Input: part model. Units: mm. Frame: model coordinates. Face numbers are marked on the shaded views. A direction names the side the tool comes from. Give positions to 0.01 mm unless a question says otherwise; leave off trailing zeros. Write each loop counter-clockwise with the first axis right and the second up, starting at its lowest first coordinate (ties: lowest second). Pieces come first, ordered by that corner, then holes. Notation, with made-up numbers: (-20.5, 2) - (-13.5, 2) arc R23 cw to (-13.5, 14) - close; hole circle Ø8 at (86.5, -12). An arc over 180 degrees is marked (long way). Use a Markdown table: item, result. Add a question column.
1. Mould query, pull axis Y, two halves, no side actions, for the marked faces 1, 2, 3 and 4. Classes: released by +Y, released by -Y, zero draft, split by the parting line, or undercut.
2. Material intervals for probe 1 along X at (y, z) = (49, -14); probe 2 along Y at (x, z) = (78.5, 1); probe 3 along Z at (x, y) = (32.5, 46), sorted ascending.
3. Section query C-C, the plane z = -5.5. Return loops of the section in (x, y).
4. Pin query (flat end, axial travel): pin 1 (1.5 mm diameter, centred on x = 49.5, y = 40, fed in from +Z); pin 2 (1 mm diameter, centred on x = 102.5, y = 47.5, fed in from -Z); pin 3 (12 mm diameter, centred on x = 31, z = -10.5, fed in from +Y). Return the tip coordinate at first contact, or that it passes through.
5. Section query B-B, the plane x = 82. Return loops of the section in (y, z), plus the area to 3 significant figures.
6. Set-up query: the marked faces 5, 6 and 7. Return all of +Z, -Z, +X, -X, +Y, -Y with unobstructed straight access to the full face (end or side cutting, diameter ignored); none if empty.
7. Section query D-D, the plane x = 6. Return loops of the section in (y, z).
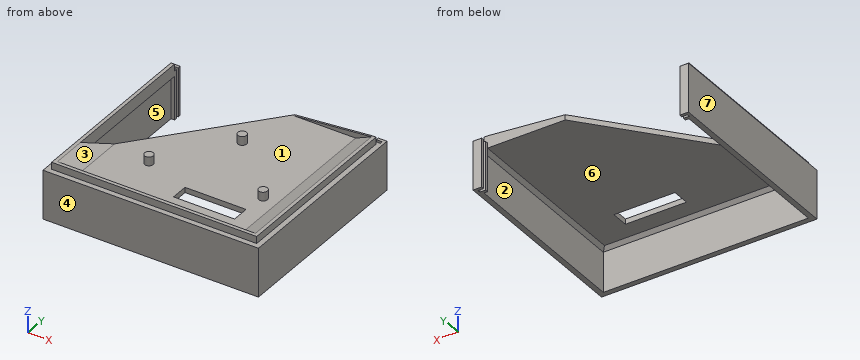
Autodesk Fusion 360 part; units mm, degrees
sketch "Sketch1" plane through (0, 0, 0) normal (0, 0, 1) x (1, 0, 0)
  line L0 (0, 0) -> (113.6, 0)
  line L1 (113.6, 0) -> (113.6, 101.8)
  line L2 (113.6, 101.8) -> (0, 101.8)
  line L3 (0, 101.8) -> (0, 0)
  line L4 (-2, -2) -> (115.6, -2)
  line L5 (115.6, -2) -> (115.6, 103.8)
  line L6 (115.6, 103.8) -> (-2, 103.8)
  line L7 (-2, 103.8) -> (-2, -2)
  line L8 (-5, -5) -> (118.6, -5)
  line L9 (118.6, -5) -> (118.6, 106.8)
  line L10 (118.6, 106.8) -> (-5, 106.8)
  line L11 (-5, 106.8) -> (-5, -5)
  dimension "d1" = 113.6
  dimension "d2" = 101.8
  dimension "d3" = 2
  dimension "d4" = 5
extrude "Extrude1" add sketch "Sketch1" along normal blind 3 contours L0 L1 L2 L3
extrude "Extrude2" add sketch "Sketch1" along normal blind 7 contours L4 L5 L6 L7
extrude "Extrude3" add sketch "Sketch1" along normal blind 3 and the other way blind 25 contours L8 L9 L10 L11
sketch "Sketch2" plane through (0, 0, 3) normal (0, 0, 1) x (-1, 0, 0)
  line L0 (0, -101.8) -> (0, 0)
  line L1 (0, 0) -> (-113.6, 0)
  line L2 (-113.6, 0) -> (-113.6, -101.8)
  line L3 (-113.6, -101.8) -> (0, -101.8)
  line L4 (-69, -101.8) -> (0, -20)
  circle A0 centre (-61.3997, -67.6905) radius 2.5
  circle A1 centre (-61.3997, -67.6905) radius 2.5
  circle A2 centre (-96.3997, -32.6905) radius 2.5
  circle A3 centre (-33.8997, -28.1905) radius 2.5
  circle A4 centre (-33.8997, -28.1905) radius 2.5
  circle A5 centre (-96.3997, -32.6905) radius 2.5
  dimension "d15" = 5
  dimension "d16" = 34.1095
  dimension "d17" = 7.6003
  dimension "d18" = 44.6
  dimension "d19" = 20
  dimension "d20" = 5
  dimension "d21" = 5
  dimension "d22" = 17.2003
  dimension "d23" = 69.1095
  dimension "d24" = 33.8997
  dimension "d25" = 28.1905
extrude "Extrude4" cut sketch "Sketch2" against normal blind 3 contours L0 L3 L4
extrude "Extrude5" add sketch "Sketch2" along normal blind 5 contours A0 A1 | A2 A5 | A3 A4
sketch "Sketch3" plane through (0, 101.8, 0) normal (0, -1, 0) x (1, 0, 0)
  line L0 (69, 3) -> (113.6, 3)
  line L1 (113.6, 3) -> (113.6, 7)
  line L2 (113.6, 7) -> (0, 7)
  line L3 (0, 7) -> (0, 0)
  line L4 (0, 0) -> (69, 0)
  line L5 (69, 0) -> (69, 3)
  line L6 (69, 3) -> (113.6, 7)
extrude "Extrude6" add sketch "Sketch3" along normal blind 1 contours L0 L1 L6
sketch "Sketch4" plane through (0, 0, 3) normal (0, 0, 1) x (-1, 0, 0)
  line L0 (-69, -100.8) -> (-69, -101.8)
  line L1 (-69, -101.8) -> (0, -20)
  line L2 (0, -20) -> (0, 0)
  line L3 (0, 0) -> (-113.6, 0)
  line L4 (-113.6, 0) -> (-113.6, -100.8)
  line L5 (-113.6, -100.8) -> (-69, -100.8)
  circle A0 centre (-96.3997, -32.6905) radius 2.5
  circle A1 centre (-33.8997, -28.1905) radius 2.5
  circle A2 centre (-61.3997, -67.6905) radius 2.5
  line L6 (-95, -20) -> (-60, -20)
  line L7 (-60, -20) -> (-60, -10)
  line L8 (-60, -10) -> (-95, -10)
  line L9 (-95, -10) -> (-95, -20)
  dimension "d34" = 18.6
  dimension "d35" = 10
  dimension "d36" = 35
  dimension "d37" = 10
extrude "Extrude7" cut sketch "Sketch4" against normal blind 3 contours L6 L7 L8 L9
extrude "Extrude8" cut 1 faces at (77.4, 106.8, -15.6667) along direction (0, -1, 0) blind 5
extrude "Extrude9" cut 1 faces at (76.4, 103.8, 4.3333) along direction (0, -1, 0) blind 2
chamfer "Chamfer1" distance 2 angle 45 3 edges at (115.6, 49.9, 0) (56.8, -2, 0) (-2, 49.9, 0)
chamfer "Chamfer2" distance 9 distance2 4 1 edges at (113.6, 50.4, 3) measured on face at (91.362, 67.8914, 3)
chamfer "Chamfer3" distance 11 distance2 4 1 edges at (0, 10, 3) measured on face at (88.3626, 67.8914, 3)
sketch "Sketch6" plane through (0, 0, 7) normal (0, 0, 1) x (-1, 0, 0)
  line L0 (0, -101.8) -> (2, -101.8)
  line L1 (2, -101.8) -> (2, 2)
  line L2 (2, 2) -> (-115.6, 2)
  line L3 (-115.6, 2) -> (-115.6, -101.8)
  line L4 (-115.6, -101.8) -> (-113.6, -101.8)
  line L5 (-113.6, -101.8) -> (-113.6, -100.8)
  line L6 (-113.6, -100.8) -> (-113.6, 0)
  line L7 (-113.6, 0) -> (0, 0)
  line L8 (0, 0) -> (0, -20)
  line L9 (0, -20) -> (0, -101.8)
  line L10 (-118.6, -101.8) -> (-113.6, -101.8)
  line L11 (-113.6, -106.8) -> (-118.6, -106.8)
  line L12 (-118.6, -106.8) -> (-118.6, -101.8)
  line L13 (-113.6, -103.5) -> (-116.9, -103.5)
  line L14 (-116.9, -103.5) -> (-116.9, -105.1)
  line L15 (-116.9, -105.1) -> (-113.6, -105.1)
  line L16 (-113.6, -101.8) -> (-113.6, -103.5)
  line L17 (-113.6, -105.1) -> (-113.6, -106.8)
  line L18 (0, -101.8) -> (5, -101.8)
  line L19 (5, -101.8) -> (5, -106.8)
  line L20 (5, -106.8) -> (0, -106.8)
  line L21 (0, -103.5) -> (3.3, -103.5)
  line L22 (3.3, -103.5) -> (3.3, -105.1)
  line L23 (3.3, -105.1) -> (0, -105.1)
  line L24 (0, -106.8) -> (0, -105.1)
  line L25 (0, -103.5) -> (0, -101.8)
  dimension "d49" = 5
  dimension "d50" = 5
  dimension "d51" = 1.6
  dimension "d52" = 1.7
  dimension "d53" = 1.7
  dimension "d54" = 5
  dimension "d55" = 5
  dimension "d56" = 1.6
  dimension "d57" = 1.7
  dimension "d58" = 1.7
extrude "Extrude10" add sketch "Sketch6" against normal blind 32 contours L0 L18 L19 L20 L21 L22 L23 L24 L25 | L4 L10 L11 L12 L13 L14 L15 L16 L17
extrude "Extrude11" cut sketch "Sketch6" against normal blind 4 contours L0 L18 L19 L20 L21 L22 L23 L24 L25 | L4 L10 L11 L12 L13 L14 L15 L16 L17
Result sheet:
| question | item | result |
|---|---|---|
| 1 | face 1 | undercut |
| 1 | face 2 | undercut |
| 1 | face 3 | zero draft |
| 1 | face 4 | released by -Y |
| 2 | probe 1 | x = -5 to -2, 115.6 to 118.6 |
| 2 | probe 2 | y = -5 to 10, 20 to 101.8 |
| 2 | probe 3 | z = 0 to 3 |
| 3 | outline | (-5, -5) - (118.6, -5) - (118.6, 106.8) - (113.6, 106.8) - (113.6, 105.1) - (116.9, 105.1) - (116.9, 103.5) - (113.6, 103.5) - (113.6, 101.8) - (115.6, 101.8) - (115.6, -2) - (-2, -2) - (-2, 101.8) - (0, 101.8) - (0, 103.5) - (-3.3, 103.5) - (-3.3, 105.1) - (0, 105.1) - (0, 106.8) - (-5, 106.8) - close |
| 4 | pin 1 | stops at z = 3 |
| 4 | pin 2 | stops at z = 0 |
| 4 | pin 3 | stops at y = -2 |
| 5 | outline | (-5, -25) - (-2, -25) - (-2, -2) - (0, 0) - (10, 0) - (10, 3) - (0, 3) - (0, 7) - (-2, 7) - (-2, 3) - (-5, 3) - close; (20, 0) - (101.8, 0) - (101.8, 4.17) - (100.8, 4.17) - (100.8, 3) - (20, 3) - close |
| 5 | area | 377 mm² |
| 6 | face 5 | -Z |
| 6 | face 6 | -Z, +Y |
| 6 | face 7 | +Z, -Z, -X, +Y, -Y |
| 7 | outline | (-5, -25) - (-2, -25) - (-2, -2) - (0, 0) - (27.11, 0) - (27.11, 4.82) - (0, 4.82) - (0, 7) - (-2, 7) - (-2, 3) - (-5, 3) - close |
